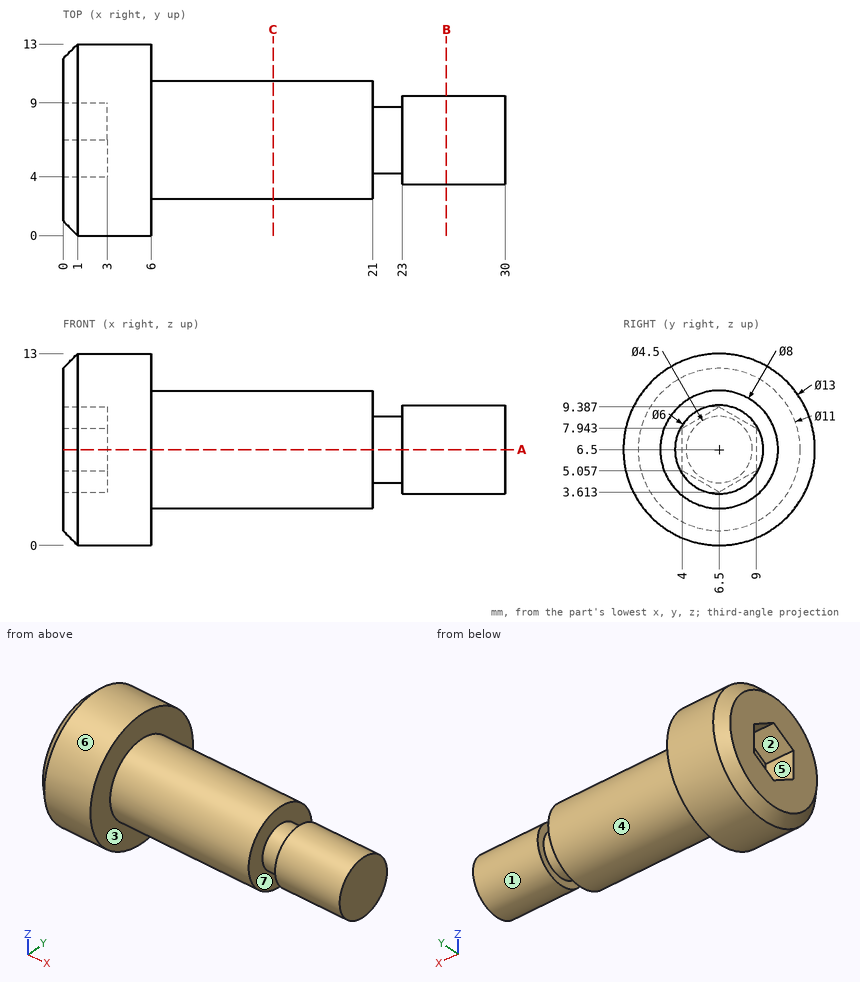
Answer from the drawing. Dimensions are ordinates in mm from the lowest x, y and z of the part. A direction names the side the tool comes from. Coordinates: 2 decimals unless noted, no trailing zeros. Loops run counter-clockwise (first coordinate to the right, second up) from the corner with the lowest first, then second, coordinate; pieces in that order, holes last.
Q1. The part is cut by section C-C on x = 14.25. Write down the section's boundary in (y, z).
Q2. The part is cut by section A-A on z = 6.5. Write down the section's boundary in (x, y).
Q3. Each of these flat-tipped pins is pushed along its axis until it touches: pin 1 Ø2.5 at (y, z) = (6.5, 5.5) entering from -X; pin 2 Ø1 at (x, z) = (20.5, 4.5) entering from -Y; pin 3 Ø6.5 at (y, z) = (7, 6) entering from -X; pin 4 Ø3 at (x, y) = (21, 11.5) entering from +Z (1 decimal). Where does it stop, or does it pass through?
Q4. Consider probe 1 along X at (y, z) = (5.75, 8.75); probe 2 along X at (y, z) = (9.75, 7.5); probe 3 along Z at (x, y) = (1.75, 5.75) (1 decimal). Determine where each line is inside the solid, lowest interval first.
Q5. The part is cut by section B-B on x = 26. Write down the section's boundary in (y, z), and give its area (3 significant figures).
Q6. The mould has two halves that part along Z. Classify the marked faces 1, 2 and 3: +Z half, -Z half, draft (parallel to the pull), parting line (faces both ways), or undercut.
Q7. Which of the six approach directions +Z, -Z, +X, -X, +Y, -Y give full straight-line access (tool end or side, diameter ignored) to the marked faces 4, 5, 6 and 7?
Results below:
1. outline: circle Ø8 at (6.5, 6.5)
2. outline: (0, 1) - (1, 0) - (6, 0) - (6, 2.5) - (21, 2.5) - (21, 4.25) - (23, 4.25) - (23, 3.5) - (30, 3.5) - (30, 9.5) - (23, 9.5) - (23, 8.75) - (21, 8.75) - (21, 10.5) - (6, 10.5) - (6, 13) - (1, 13) - (0, 12) - (0, 9) - (3, 9) - (3, 4) - (0, 4) - close
3. pin 1: stops at x = 3
3. pin 2: stops at y = 2.79
3. pin 3: stops at x = 0
3. pin 4: stops at z = 8.4
4. probe 1: x = 3 to 21, 23 to 30
4. probe 2: x = 0 to 21
4. probe 3: z = 0 to 4, 9 to 13
5. outline: circle Ø6 at (6.5, 6.5)
5. area: 28.3 mm2
6. face 1: parting line
6. face 2: undercut
6. face 3: draft
7. face 4: +X
7. face 5: -X
7. face 6: +X, -X
7. face 7: none
